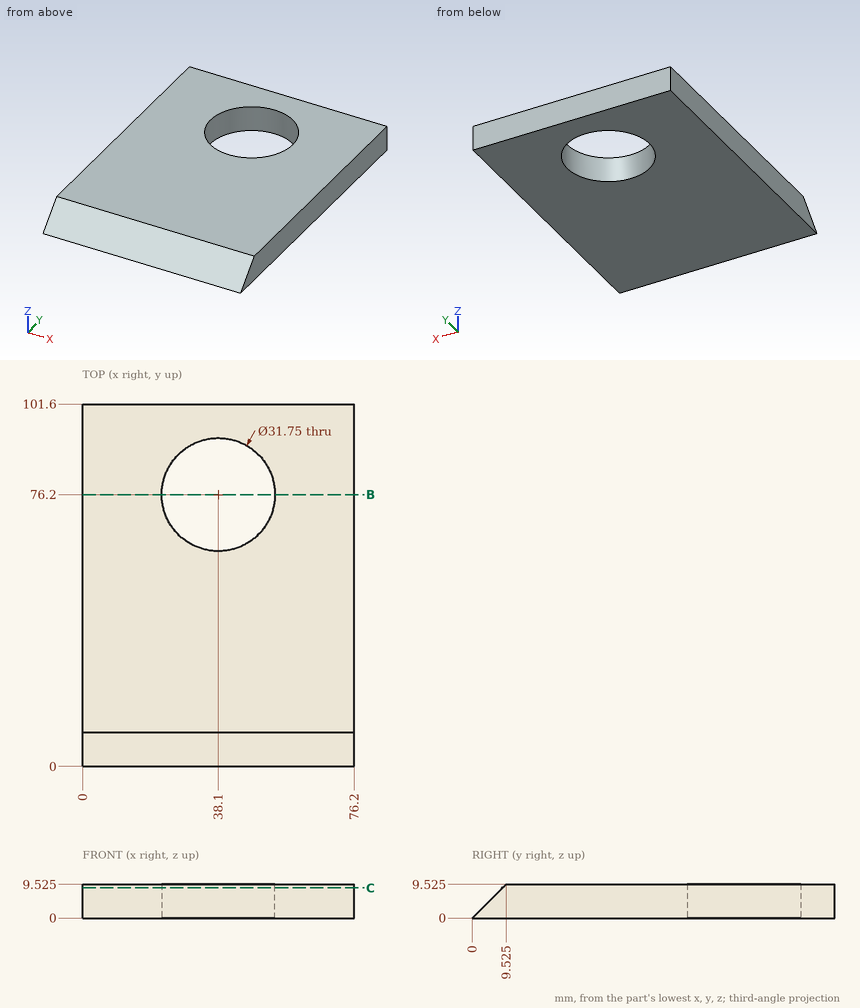
Verification items for this drawing (mm, ordinates from the low corner). Round coordinates to 2 decimals unless told otherwise and drop trailing zeros. Write each loop counter-clockwise with the first axis right and the second up, starting at its lowest first coordinate (ties: lowest second). Pieces come first, ordered by that corner, then holes. Notation, with made-up numbers: M -16,73.25 L 34,73.25 A15 ccw 34,88.25 Z; hole C 27,42.25 d8. An arc over 180 degrees is marked long. Write item = value, one per line. Start each with the question number.
1. Gauge pin test, flat ends, axial feed: pin 1 (1.5 mm diameter, centred on x = 61, z = 7.5, fed in from -Y); pin 2 (3 mm diameter, centred on x = 59.5, z = 6, fed in from -Y). Record the tip position at first contact, or that the pin passes through.
2. Section check B-B, the plane y = 76.2. Record the cut outline in (x, z) (3 decimals), then the cut area to 3 significant figures.
3. Section check C-C, the plane z = 8.5. Record the cut outline in (x, y) (3 decimals).
4. Scan lines: line 1 (X direction, y = 76.2, z = 7.5) (3 decimals); line 2 (Y direction, x = 38.1, z = 2.75) (3 decimals); line 3 (X direction, y = 74, z = 1.5). Record each from-to range of solid material in increasing order. Write a range as [from, to].
Results found:
q1.pin_1 = 6.75
q1.pin_2 = 4.5
q2.outline = M 0,0 L 22.225,0 L 22.225,9.525 L 0,9.525 Z; M 53.975,0 L 76.2,0 L 76.2,9.525 L 53.975,9.525 Z
q2.area = 423 mm^2
q3.outline = M 0,8.5 L 76.2,8.5 L 76.2,101.6 L 0,101.6 Z; hole C 38.1,76.2 d31.75
q4.line_1 = [0, 22.225], [53.975, 76.2]
q4.line_2 = [2.75, 60.325], [92.075, 101.6]
q4.line_3 = [0, 22.38], [53.82, 76.2]
